Autodesk Fusion 360 part; units mm, degrees
sketch "Sketch1" plane through (0, 0, 0) normal (0, 0, 1) x (1, 0, 0)
sketch "Sketch3" plane through (0, 0, 0) normal (0, 0, 1) x (1, 0, 0)
  line L0 (0, 0) -> (66, 0)
  line L1 (66, 0) -> (66, 42)
  line L2 (66, 42) -> (0, 42)
  line L3 (0, 42) -> (0, 0)
  line L4 (66, 0) -> (54, 0)
  line L5 (54, 0) -> (54, 12)
  line L6 (54, 12) -> (66, 12)
  line L7 (66, 12) -> (66, 0)
  line L8 (66, 42) -> (54, 42)
  line L9 (54, 42) -> (54, 30)
  line L10 (54, 30) -> (66, 30)
  line L11 (66, 30) -> (66, 42)
  line L12 (54, 42) -> (66, 30)
  line L13 (66, 12) -> (54, 0)
  point P0 (54, 42)
  point P1 (66, 30)
  point P2 (54, 0)
  point P3 (66, 12)
  dimension "d11" = 66
  dimension "d12" = 42
  dimension "d13" = 12
  dimension "d14" = 12
  dimension "d15" = 12
  dimension "d16" = 12
extrude "Extrude1" add sketch "Sketch3" along normal blind 12 contours L0 L1 L2 L3 L5 L6 L9 L10 | L5 L6 L13 | L9 L10 L12
sketch "Sketch4" plane through (0, 0, 0) normal (1, 0, 0) x (0, 1, 0)
  line L0 (0, 0) -> (42, 0)
  line L1 (42, 0) -> (42, 39)
  line L2 (21.0001, 60) -> (21, 60)
  line L3 (0, 39) -> (0, 0)
  line L4 (21, 0) -> (21, 39)
  line L5 (0, 39) -> (42, 39)
  arc A0 (21, 60) -> (0, 39) centre (21, 39) ccw
  arc A1 (42, 39) -> (21.0001, 60) centre (21, 39) ccw
  point P0 (0, 60)
  dimension "d19" = 42
  dimension "d20" = 60
  dimension "d21" = 39
  dimension "d22" = 21
extrude "Extrude2" add sketch "Sketch4" along normal blind 12
sketch "Sketch5" plane through (0, 0, 12) normal (0, 0, 1) x (-1, 0, 0)
  line L0 (-12, -42) -> (-12, 0)
  line L1 (-12, 0) -> (-54, 0)
  line L2 (-54, 0) -> (-66, -12)
  line L3 (-66, -12) -> (-66, -30)
  line L4 (-66, -30) -> (-54, -42)
  line L5 (-54, -42) -> (-12, -42)
  line L6 (-25, 0) -> (-25, -15)
  line L7 (-25, -27) -> (-25, -42)
  line L8 (-25, -42) -> (-25, -27)
  line L9 (-12, -27) -> (-66, -27)
  line L10 (-66, -27) -> (-66, -15)
  line L11 (-66, -15) -> (-12, -15)
  line L12 (-12, -15) -> (-12, -27)
  dimension "d25" = 15
  dimension "d26" = 15
  dimension "d27" = 15
  dimension "d28" = 12
extrude "Extrude3" add sketch "Sketch5" along normal blind 42 contours L0 L3 L9 L10 L11 L12
sketch "Sketch6" plane through (0, 15, 0) normal (0, -1, 0) x (1, 0, 0)
  line L0 (12, 12) -> (66, 12)
  line L1 (66, 12) -> (66, 54)
  line L2 (66, 54) -> (12, 54)
  line L3 (12, 54) -> (12, 12)
  line L4 (66, 12) -> (12, 54)
extrude "Extrude4" cut sketch "Sketch6" against normal blind 29 contours L1 L2 L4
sketch "Sketch7" plane through (30.6923, 0, 39.4615) normal (0.6139, 0, 0.7894) x (0, 1, 0)
  line L0 (27, -44.73) -> (27, 23.6806)
  line L1 (27, 23.6806) -> (15, 23.6806)
  line L2 (15, 23.6806) -> (15, -44.73)
  line L3 (15, -44.73) -> (27, -44.73)
  dimension "d33" = 12
sketch "Sketch2" plane through (0, 0, 0) normal (1, 0, 0) x (0, 1, 0)
  line L0 (0, 0) -> (42, 0)
  line L1 (42, 0) -> (42, 60)
  line L2 (42, 60) -> (0, 60)
  line L3 (0, 60) -> (0, 0)
  dimension "d5" = 60
  dimension "d6" = 42
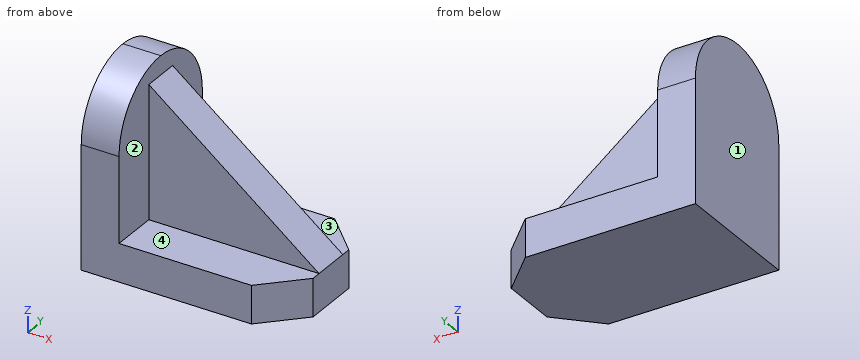
Verification items for the finished model (mm, model axes). Face numbers are marked on the shaded views. A direction names the side the tool comes from. Coordinates: 2 decimals unless noted, no trailing zeros. Write each loop counter-clockwise with the first axis right and the second up, starting at its lowest first coordinate (ties: lowest second). Pieces come first, ordered by that corner, then holes. Notation, with made-up numbers: (-14.75, 51) - (21.25, 51) arc R29 cw to (21.25, 75) - close; hole circle Ø6 at (56, -34.75). An arc over 180 degrees is marked (long way). Answer as a JSON object with one key per item and string values.
(1) Cross-section at D-D on x = 5.5. Record the cut outline in (y, z), plus the area to 3 significant figures.
Report:
{"outline": "(0, 0) - (42, 0) - (42, 39) arc R21 ccw to (0, 39) - close", "area": "2,330 mm^2"}
(2) Cross-section at C-C on y = 33. Record the cut outline in (x, z).
Report:
{"outline": "(0, 0) - (63, 0) - (63, 12) - (12, 12) - (12, 56.23) - (0, 56.23) - close"}
(3) Thickness scan on line 1 along X through (y, z) = (7.5, 42.5); line 2 along Y through (x, z) = (38, 30). Record the ranges inside material, lowest first.
Report:
{"line 1": "0 to 12", "line 2": "15 to 27"}
(4) Tool access check on the marked faces 1, 2, 3 and 4. Record the directions out of +Z, -Z, +X, -X, +Y, -Y that give a thin tool (end or side, any length) a straight path to the whole face; none if there is none.
Report:
{"face 1": "+Z, -Z, -X, +Y, -Y", "face 2": "+Z, +X", "face 3": "+Z, +X, +Y", "face 4": "+Z, +X, -Y"}
(5) Gauge pin test, flat ends, axial feed: pin 1 Ø12 at (x, y) = (31.5, 31.5) entering from +Z; pin 2 Ø10 at (x, z) = (38.5, 36) entering from +Y; pin 3 Ø12.5 at (y, z) = (21, 35.5) entering from +X. Record the tip position at first contact, or that the pin passes through.
Report:
{"pin 1": "z = 41.92", "pin 2": "y = 27", "pin 3": "x = 43.82"}
(6) Cross-section at A-A on x = 25.5. Record the cut outline in (y, z).
Report:
{"outline": "(0, 0) - (42, 0) - (42, 12) - (27, 12) - (27, 43.5) - (15, 43.5) - (15, 12) - (0, 12) - close"}
(7) Cross-section at B-B on z = 23. Record the cut outline in (x, y), plus the area to 3 significant figures.
Report:
{"outline": "(0, 0) - (12, 0) - (12, 15) - (51.86, 15) - (51.86, 27) - (12, 27) - (12, 42) - (0, 42) - close", "area": "982 mm^2"}
